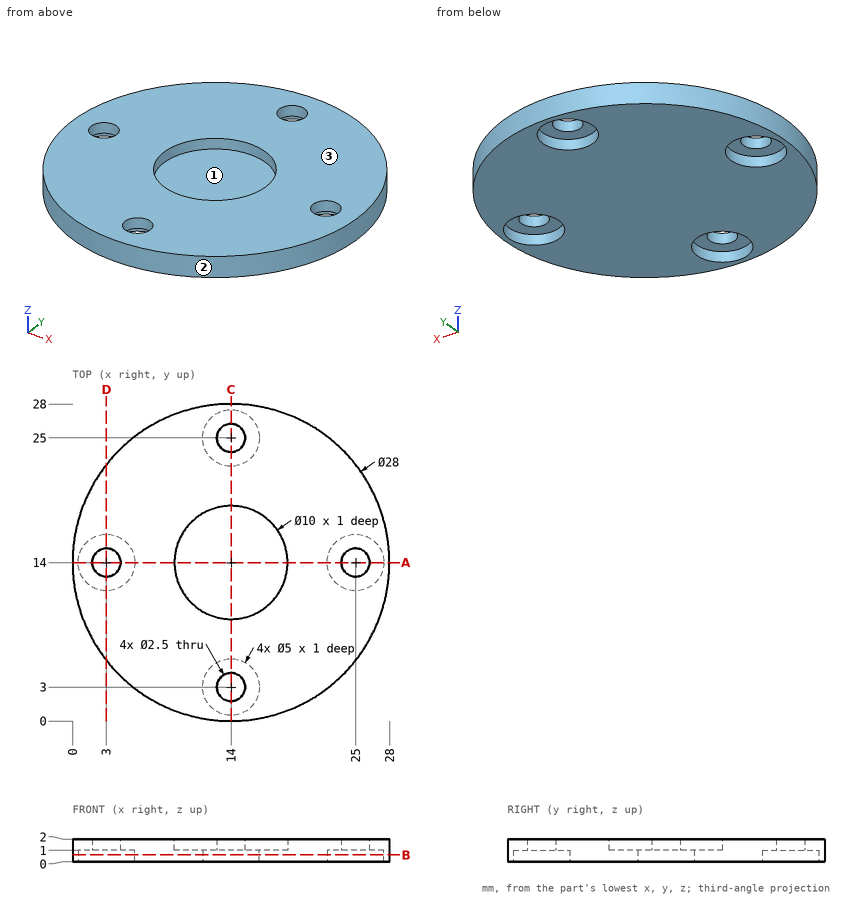
Drawing for the job (mm, zero at the part's lowest x, y, z). Round coordinates to 2 decimals unless told otherwise and drop trailing zeros. Loops run counter-clockwise (first coordinate to the right, second up) from the corner with the lowest first, then second, coordinate; pieces in that order, holes last. Notation, with made-up numbers: (-17, 75) -> (23, 75) arc R4 cw to (23, 81) -> close; hole circle Ø2 at (33.5, -37). An arc over 180 degrees is marked (long way). Use one line per item in the form item = value. Start each with the question number.
Item 1: Drill centre lines: line 1 along Y through (x, z) = (14, 0.55); line 2 along Y through (x, z) = (14, 1.65); line 3 along Y through (x, z) = (15.5, 0.95). Where is each one in solid material? Low to high.
Item 2: Drop flat-ended pins along their axis: pin 1 Ø4 at (x, y) = (25, 14) entering from -Z; pin 2 Ø1 at (y, z) = (25, 1) entering from -X; pin 3 Ø9 at (x, y) = (14, 14) entering from +Z. Give the stop position or say it passes through.
Item 3: Two-plate mould, pull along Y, no slides. Class the marked faces 1, 2 and 3: released by +Y, released by -Y, zero draft, split by the parting line, or undercut.
Item 4: Band-saw the part on A-A (y = 14). List the corners of the cut face in (x, z).
Item 5: Band-saw the part on B-B (z = 0.6). List the corners of the cut face in (x, y).
Item 6: Band-saw the part on D-D (x = 3). List the corners of the cut face in (y, z).
Data:
q1.line_1 = 0 to 0.5, 5.5 to 22.5, 27.5 to 28
q1.line_2 = 0 to 1.75, 4.25 to 9, 19 to 23.75, 26.25 to 28
q1.line_3 = 0.08 to 1, 5 to 23, 27 to 27.92
q2.pin_1 = 1
q2.pin_2 = 4.74
q2.pin_3 = 1
q3.face_1 = undercut
q3.face_2 = split by the parting line
q3.face_3 = zero draft
q4.outline = (0, 0) -> (0.5, 0) -> (0.5, 1) -> (1.75, 1) -> (1.75, 2) -> (0, 2) -> close; (4.25, 1) -> (5.5, 1) -> (5.5, 0) -> (22.5, 0) -> (22.5, 1) -> (23.75, 1) -> (23.75, 2) -> (19, 2) -> (19, 1) -> (9, 1) -> (9, 2) -> (4.25, 2) -> close; (26.25, 1) -> (27.5, 1) -> (27.5, 0) -> (28, 0) -> (28, 2) -> (26.25, 2) -> close
q5.outline = circle Ø28 at (14, 14); hole circle Ø5 at (3, 14); hole circle Ø5 at (14, 3); hole circle Ø5 at (14, 25); hole circle Ø5 at (25, 14)
q6.outline = (5.34, 0) -> (11.5, 0) -> (11.5, 1) -> (12.75, 1) -> (12.75, 2) -> (5.34, 2) -> close; (15.25, 1) -> (16.5, 1) -> (16.5, 0) -> (22.66, 0) -> (22.66, 2) -> (15.25, 2) -> close
